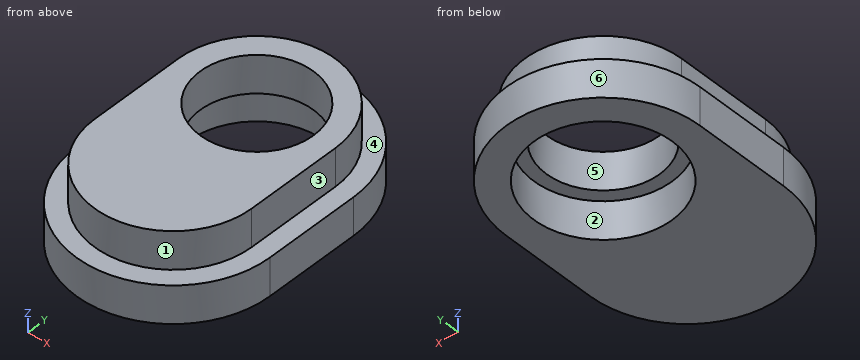
```python
from build123d import *

# Parameters (mm, degrees)
SKETCH1_R           = 4.5
BOSS_EXTRUDE1_DEPTH = 6
SKETCH3_R           = 5.5
BOSS_EXTRUDE2_DEPTH = 3
SKETCH4_R           = 5.5
CUT_EXTRUDE1_DEPTH  = 3


with BuildPart() as part:
    # Sketch1 → Boss-Extrude1 (new body)
    with BuildSketch(Plane.XY):
        with BuildLine():
            Line((6.25, 0), (6.25, -7.5))
            ThreePointArc((6.25, -7.5), (0, -13.75), (-6.25, -7.5))
            Line((-6.25, -7.5), (-6.25, 0))
            ThreePointArc((-6.25, 0), (0, 6.25), (6.25, 0))
        make_face()
        Circle(SKETCH1_R, mode=Mode.SUBTRACT)
    extrude(amount=BOSS_EXTRUDE1_DEPTH)

    # Sketch3 → Boss-Extrude2 (add)
    with BuildSketch(Plane(origin=(0, 0, 0), x_dir=(-1, 0, 0), z_dir=(0, 0, -1))):
        with BuildLine():
            Line((7.7, 0), (7.7, -7.5))
            ThreePointArc((7.7, -7.5), (0, -15.2), (-7.7, -7.5))
            Line((-7.7, -7.5), (-7.7, 0))
            ThreePointArc((-7.7, 0), (0, 7.7), (7.7, 0))
        make_face()
        Circle(SKETCH3_R, mode=Mode.SUBTRACT)
    extrude(amount=-BOSS_EXTRUDE2_DEPTH)

    # Sketch4 → Cut-Extrude1 (cut)
    with BuildSketch(Plane(origin=(0, 0, 0), x_dir=(-1, 0, 0), z_dir=(0, 0, -1))):
        Circle(SKETCH4_R)
    extrude(amount=-CUT_EXTRUDE1_DEPTH, mode=Mode.SUBTRACT)


solid = part.part
```
Here's how the part is built. I have some questions about the finished solid (model axes, mm). Face numbers are marked on the shaded views. A direction names the side the tool comes from. Give positions to 0.01 mm unless a question says otherwise; leave off trailing zeros. Loops run counter-clockwise (first coordinate to the right, second up) from the corner with the lowest first, then second, coordinate; pieces in that order, holes last. Notation, with made-up numbers: M 61.25,83.5 L 105.25,83.5 A20 cw 105.25,114.5 Z; hole C 63.5,51 d3. An arc over 180 degrees is marked long. Use one line per item in the form item = value. Start each with the question number.
Q1. If we section it at D-D (x = -5.75): Write out the boundary of the cut face in (y, z), then the cut area to 3 significant figures.
Q2. Which directions (+Z, -Z, +X, -X, +Y, -Y) give clear straight access to the entire face, cutting with the end or side of a thin tool? Please do the marked faces 1, 2 and 3.
Q3. If we section it at B-B (y = 3.5): Write out the boundary of the cut face in (x, z).
Q4. Will these pins go through, and if not, where does the flat tip stop? pin 1 Ø5.5 at (x, y) = (0, -2) entering from -Z; pin 2 Ø1.5 at (x, z) = (-2, 2) entering from +Y; pin 3 Ø0.9 at (y, z) = (-3, 5) entering from -X.
Q5. If we section it at C-C (z = 5.4): Write out the boundary of the cut face in (x, y), then the cut area to 3 significant figures.
Q6. I need wall thicknesses on line 1 along Y through (x, z) = (0, 5.15); line 2 along X through (y, z) = (2.5, 1.4); line 3 along Z through (x, y) = (-2.25, -14). Which ranges of each line are inside material? Lowest first, please.
Q7. If we section it at A-A (x = 0): Write out the boundary of the cut face in (y, z).
Q8. Thinking about a two-plate mould opening in X: for the marked faces 4, 5 and 6, which applies, +X half, -X half, draft (parallel to the pull), parting line (faces both ways), or undercut?
Taken from the geometry:
q1.outline = M -12.62,0 L 5.12,0 L 5.12,3 L 2.45,3 L 2.45,6 L -9.95,6 L -9.95,3 L -12.62,3 Z
q1.area = 90.4 mm^2
q2.face_1 = +Z, -Y
q2.face_2 = -Z
q2.face_3 = +Z, +X, +Y, -Y
q3.outline = M -6.86,0 L -4.24,0 L -4.24,3 L -2.83,3 L -2.83,6 L -5.18,6 L -5.18,3 L -6.86,3 Z; M 2.83,3 L 4.24,3 L 4.24,0 L 6.86,0 L 6.86,3 L 5.18,3 L 5.18,6 L 2.83,6 Z
q4.pin_1 = 3
q4.pin_2 = 7.6
q4.pin_3 = -6.25
q5.outline = M -6.25,-7.5 A6.25 ccw 6.25,-7.5 L 6.25,0 A6.25 ccw -6.25,0 Z; hole C 0,0 d9
q5.area = 153 mm^2
q6.line_1 = -13.75 to -4.5, 4.5 to 6.25
q6.line_2 = -7.28 to -4.9, 4.9 to 7.28
q6.line_3 = 0 to 3
q7.outline = M -15.2,0 L -5.5,0 L -5.5,3 L -4.5,3 L -4.5,6 L -13.75,6 L -13.75,3 L -15.2,3 Z; M 4.5,3 L 5.5,3 L 5.5,0 L 7.7,0 L 7.7,3 L 6.25,3 L 6.25,6 L 4.5,6 Z
q8.face_4 = draft
q8.face_5 = undercut
q8.face_6 = parting line
